```python
from build123d import *

# Parameters (mm, degrees)
F0_R     = 6.35
F1_DEPTH = 2.54
F3_R     = 3.175
F4_DEPTH = 7.9375


# Not quite as in the source:
# - a fillet or chamfer that OpenCascade refuses, or shapes differently, is made with other operations: its cross-section is extruded or revolved along the edge and cut away or added


with BuildPart() as f1:
    # F0 (on Top) → F1 (new body)
    with BuildSketch(Plane.XY):
        Circle(F0_R)
    extrude(amount=F1_DEPTH)

    # F2: fillet of radius 3.0660512242 on 1 edges, made by hand

    # F2_s1 → F2_t2 (revolve, cut)
    with BuildSketch(Plane.XZ):
        with BuildLine():
            ThreePointArc((6.35, 0), (5.3027068749, 1.8206027884), (3.3294139279, 2.54))
            Line((3.3294139279, 2.54), (6.35, 2.54))
            Line((6.35, 2.54), (6.35, 0))
        make_face()
    revolve(axis=Axis((0, 0, 2.54), (0, 0, 1)), mode=Mode.SUBTRACT)

    # F3 (on face) → F4 (join)
    with BuildSketch(Plane(origin=(0, 0, 0), x_dir=(1, 0, 0), z_dir=(0, 0, -1))):
        Circle(F3_R)
    extrude(amount=F4_DEPTH)


solid = f1.part
```
Can you work these out from the model? Positions are in its coordinate system, mm. A direction names the side the tool comes from. Coordinates: 2 decimals unless noted, no trailing zeros. Loops run counter-clockwise (first coordinate to the right, second up) from the corner with the lowest first, then second, coordinate; pieces in that order, holes last.
1) For pin 1 (6 mm diameter, centred on x = 2, z = -3.5, fed in from +Y) (3 decimals); pin 2 (6 mm diameter, centred on y = -3.5, z = -1, fed in from +X); pin 3 (5 mm diameter, centred on y = 5, z = -6, fed in from -X); pin 4 (1 mm diameter, centred on x = -4, z = -3.5, fed in from +Y), each with a flat end and sliding along its axis, tell me the tip position at first contact or that it passes through.
2) I need wall thicknesses on probe 1 along Z at (x, y) = (-3.25, 0.25); probe 2 along X at (y, z) = (0, -1) (3 decimals); probe 3 along Z at (x, y) = (-4.75, 2). Which ranges of each line are inside material? Lowest first, please.
3) Which directions (+Z, -Z, +X, -X, +Y, -Y) give clear straight access to the entire face, cutting with the end or side of a thin tool? Please do faces 1 (the flat face through (-2, 3, 0)), 2 (the flat face through (0, 0, -7.938)).
4) Imagine slicing it at D-D on z = 1.5. List the corners of the cut face in (x, y) for me.
5) Imagine slicing it at C-C on z = -6.75. List the corners of the cut face in (x, y) for me (3 decimals).
Completed:
1. pin 1: stops at y = 3.175
1. pin 2: stops at x = 6.31
1. pin 3: stops at x = -1.96
1. pin 4: passes through
2. probe 1: z = 0 to 2.54
2. probe 2: x = -3.175 to 3.175
2. probe 3: z = 0 to 1.94
3. face 1: -Z
3. face 2: -Z, +X, -X, +Y, -Y
4. outline: circle Ø11.26 at (0, 0)
5. outline: circle Ø6.35 at (0, 0)
